Here's how the part is built. I have some questions about the finished solid (model axes, mm). Give positions to 0.01 mm unless a question says otherwise; leave off trailing zeros. Loops run counter-clockwise (first coordinate to the right, second up) from the corner with the lowest first, then second, coordinate; pieces in that order, holes last.
Q1. I need wall thicknesses on probe 1 along Y at (x, z) = (92, 177.8); probe 2 along Y at (x, z) = (-84, 69); probe 3 along X at (y, z) = (-22, 156). Which ranges of each line are inside material? Lowest first, please.
Q2. Suppose I cut it at D-D (x = 133). List the corners of the cut face in (y, z) for me (3 decimals).
Q3. Suppose I cut it at B-B (x = 94). List the corners of the cut face in (y, z) for me (3 decimals), and give its area (3 significant figures).
Q4. Suppose I cut it at A-A (z = 207.5). List the corners of the cut face in (x, y) for me.
Q5. Suppose I cut it at C-C (y = 23.5). List the corners of the cut face in (x, z) for me.
Q6. I'm going to push flat-ended pins straight in: P1, Ø19, axis at y = 2.61, z = 177.8, coming from the -X side; P2, Ø8, axis at y = 10.5, z = 122, coming from the -X side; P3, Ø19, axis at y = 97.86, z = 69.85, coming from the +X side. Where does each tip first touch, or does it pass through?
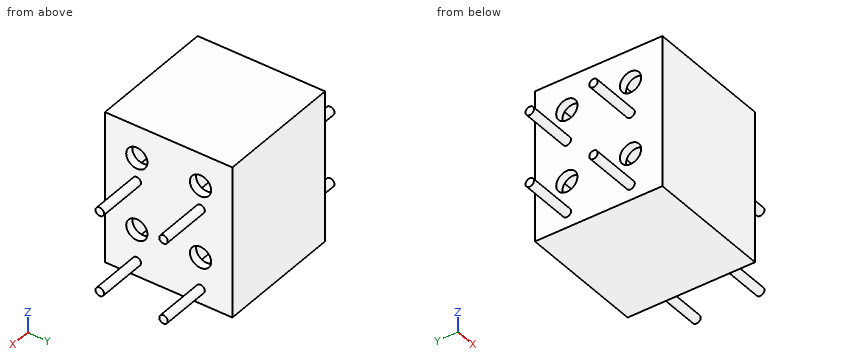
```python
from build123d import *

# Parameters (mm, degrees)
F0_W      = 177.8
F0_H      = 177.8
F1_DEPTH  = 12.7
F2_W      = 177.8
F2_H      = 203.2
F3_DEPTH  = 12.7
F4_W      = 165.1
F4_H      = 203.2
F5_DEPTH  = 12.7
F6_W      = 165.1
F6_H      = 12.7
F7_DEPTH  = 165.1
F8_W      = 12.7
F8_H      = 76.2
F8_W_2    = 76.2
F8_H_2    = 12.7
F9_DEPTH  = 203.2
F10_W     = 76.2
F10_H     = 95.25
F11_DEPTH = 12.7
F12_W     = 76.2
F12_H     = 95.25
F13_DEPTH = 12.7
F15_D     = 31.75
F15_DEPTH = 12.7
F15_TIP   = 9.5386623271
F17_D     = 31.75
F17_DEPTH = 12.7
F17_TIP   = 9.5386623271
F18_W     = 190.5
F18_H     = 190.5
F19_DEPTH = 10.414
F14_R     = 6.35
F20_DEPTH = 76.2
F16_R     = 6.35
F21_DEPTH = 76.2


with BuildPart() as f1:
    # F0 (on Top) → F1 (new body)
    with BuildSketch(Plane.XY):
        with Locations((13.2262037635, 56.5882699132)):
            Rectangle(F0_W, F0_H)
    extrude(amount=F1_DEPTH)

    # F2 (on face) → F3 (join)
    with BuildSketch(Plane.YZ.offset(102.1262037635)):
        with Locations((56.5882699132, 114.3)):
            Rectangle(F2_W, F2_H)
    extrude(amount=-F3_DEPTH)

    # F4 (on face) → F5 (join)
    with BuildSketch(Plane(origin=(0, 145.4882699132, 0), x_dir=(-1, 0, 0), z_dir=(0, 1, 0))):
        with Locations((-6.8762037635, 114.3)):
            Rectangle(F4_W, F4_H)
    extrude(amount=-F5_DEPTH)

    # F6 (on face) → F7 (join, through all)
    with BuildSketch(Plane(origin=(89.4262037635, 0, 0), x_dir=(0, -1, 0), z_dir=(-1, 0, 0))):
        with Locations((-50.2382699132, 114.3)):
            Rectangle(F6_W, F6_H)
    extrude(amount=F7_DEPTH)

    # F8 (on face) → F9 (join, through all)
    with BuildSketch(Plane.XY.offset(12.7)):
        with Locations((6.8762037635, 94.6882699132)):
            Rectangle(F8_W, F8_H)
        with Locations((-37.5737962365, 50.2382699132)):
            Rectangle(F8_W_2, F8_H_2)
        with Locations((6.8762037635, 50.2382699132)):
            Rectangle(F8_W, F8_H_2)
        with Locations((6.8762037635, 5.7882699132)):
            Rectangle(F8_W, F8_H)
        with Locations((51.3262037635, 50.2382699132)):
            Rectangle(F8_W_2, F8_H_2)
    extrude(amount=F9_DEPTH)

    # F10 (on face) → F11 (join)
    with BuildSketch(Plane(origin=(-75.6737962365, 0, 0), x_dir=(0, -1, 0), z_dir=(-1, 0, 0))):
        Polygon((-132.7882699132, 215.9), (-145.4882699132, 215.9), (-145.4882699132, 0), (32.3117300868, 0), (32.3117300868, 12.7), (-43.8882699132, 12.7), (-43.8882699132, 107.95), (32.3117300868, 107.95), (32.3117300868, 120.65), (-43.8882699132, 120.65), (-43.8882699132, 215.9), (-56.5882699132, 215.9), (-56.5882699132, 120.65), (-132.7882699132, 120.65), align=None)
        with Locations((-94.6882699132, 60.325)):
            Rectangle(F10_W, F10_H, mode=Mode.SUBTRACT)
        with Locations((-94.6882699132, 168.275)):
            Rectangle(F10_W, F10_H)
        with Locations((-5.7882699132, 168.275)):
            Rectangle(F10_W, F10_H)
        with Locations((-5.7882699132, 60.325)):
            Rectangle(F10_W, F10_H)
        with Locations((-94.6882699132, 60.325)):
            Rectangle(F10_W, F10_H)
    extrude(amount=F11_DEPTH)

    # F12 (on face) → F13 (join)
    with BuildSketch(Plane.XZ.offset(32.3117300868)):
        Polygon((-75.6737962365, 215.9), (-88.3737962365, 215.9), (-88.3737962365, 0), (102.1262037635, 0), (102.1262037635, 215.9), (89.4262037635, 215.9), (89.4262037635, 120.65), (13.2262037635, 120.65), (13.2262037635, 215.9), (0.5262037635, 215.9), (0.5262037635, 120.65), (-75.6737962365, 120.65), align=None)
        with Locations((-37.5737962365, 60.325)):
            Rectangle(F12_W, F12_H, mode=Mode.SUBTRACT)
        with Locations((51.3262037635, 60.325)):
            Rectangle(F12_W, F12_H, mode=Mode.SUBTRACT)
        with Locations((-37.5737962365, 168.275)):
            Rectangle(F12_W, F12_H)
        with Locations((51.3262037635, 168.275)):
            Rectangle(F12_W, F12_H)
        with Locations((-37.5737962365, 60.325)):
            Rectangle(F12_W, F12_H)
        with Locations((51.3262037635, 60.325)):
            Rectangle(F12_W, F12_H)
    extrude(amount=F13_DEPTH)

    # F15
    with Locations(Plane.YZ.offset(102.1262037635)):
        with Locations((2.6132699132, 177.8), (97.8632699132, 177.8), (2.6132699132, 69.85), (97.8632699132, 69.85)):
            Hole(F15_D / 2, depth=F15_DEPTH)
            with Locations((0, 0, -(F15_DEPTH + F15_TIP / 2))):  # 118° drill point
                Cone(0, F15_D / 2, F15_TIP, mode=Mode.SUBTRACT)

    # F17
    with Locations(Plane(origin=(-88.3737962365, 0, 0), x_dir=(0, -1, 0), z_dir=(-1, 0, 0))):
        with Locations((-97.8632699132, 177.8), (-2.6132699132, 177.8), (-97.8632699132, 69.85), (-2.6132699132, 69.85)):
            Hole(F17_D / 2, depth=F17_DEPTH)
            with Locations((0, 0, -(F17_DEPTH + F17_TIP / 2))):  # 118° drill point
                Cone(0, F17_D / 2, F17_TIP, mode=Mode.SUBTRACT)

    # F18 (on face) → F19 (join)
    with BuildSketch(Plane.XY.offset(215.9)):
        with Locations((6.8762037635, 50.2382699132)):
            Rectangle(F18_W, F18_H)
    extrude(amount=F19_DEPTH)

    # F14 (on face) → F20 (join)
    with BuildSketch(Plane.YZ.offset(102.1262037635)):
        with Locations((2.6132699132, 142.875)):
            Circle(F14_R)
        with Locations((2.6132699132, 22.225)):
            Circle(F14_R)
        with Locations((97.8632699132, 142.875)):
            Circle(F14_R)
        with Locations((97.8632699132, 22.225)):
            Circle(F14_R)
    extrude(amount=F20_DEPTH)

    # F16 (on face) → F21 (join)
    with BuildSketch(Plane(origin=(-88.3737962365, 0, 0), x_dir=(0, -1, 0), z_dir=(-1, 0, 0))):
        with Locations((-97.8632699132, 130.175)):
            Circle(F16_R)
        with Locations((-97.8632699132, 22.225)):
            Circle(F16_R)
        with Locations((-2.6132699132, 130.175)):
            Circle(F16_R)
        with Locations((-2.6132699132, 22.225)):
            Circle(F16_R)
    extrude(amount=F21_DEPTH)


solid = f1.part
```
Solutions:
1. probe 1: y = -45.01 to -13.26, 18.49 to 81.99, 113.74 to 145.49
1. probe 2: y = -45.01 to -13.24, 18.47 to 82.01, 113.72 to 145.49
1. probe 3: x = -88.37 to -75.67, 0.53 to 13.23, 89.43 to 102.13
2. outline: circle Ø12.7 at (2.613, 22.225); circle Ø12.7 at (2.613, 142.875); circle Ø12.7 at (97.863, 22.225); circle Ø12.7 at (97.863, 142.875)
3. outline: (-45.012, 0) - (145.488, 0) - (145.488, 226.314) - (-45.012, 226.314) - close; hole circle Ø31.75 at (2.613, 69.85); hole circle Ø31.75 at (2.613, 177.8); hole circle Ø31.75 at (97.863, 69.85); hole circle Ø31.75 at (97.863, 177.8)
3. area: 39,900 mm2
4. outline: (-88.37, -45.01) - (102.13, -45.01) - (102.13, 145.49) - (-88.37, 145.49) - close; hole (-75.67, -32.31) - (0.53, -32.31) - (0.53, 43.89) - (-75.67, 43.89) - close; hole (-75.67, 56.59) - (0.53, 56.59) - (0.53, 132.79) - (-75.67, 132.79) - close; hole (13.23, -32.31) - (89.43, -32.31) - (89.43, 43.89) - (13.23, 43.89) - close; hole (13.23, 56.59) - (89.43, 56.59) - (89.43, 132.79) - (13.23, 132.79) - close
5. outline: (-88.37, 0) - (102.13, 0) - (102.13, 226.31) - (-88.37, 226.31) - close; hole (-75.67, 12.7) - (0.53, 12.7) - (0.53, 107.95) - (-75.67, 107.95) - close; hole (-75.67, 120.65) - (0.53, 120.65) - (0.53, 215.9) - (-75.67, 215.9) - close; hole (13.23, 12.7) - (89.43, 12.7) - (89.43, 107.95) - (13.23, 107.95) - close; hole (13.23, 120.65) - (89.43, 120.65) - (89.43, 215.9) - (13.23, 215.9) - close
6. P1: stops at x = 0.53
6. P2: stops at x = -88.37
6. P3: stops at x = 13.23
